Input: part model. Units: mm. Frame: model coordinates. A direction names the side the tool comes from. Coordinates: 2 decimals unless noted, no trailing zeros. Order: outer loops, then holes, each group sorted by start corner. A loop starts at its lowest first (then second) coordinate and runs counter-clockwise, first axis right, second up.
Autodesk Fusion 360 part; units mm, degrees
sketch "Esquisse1" plane through (0, 0, 0) normal (0, 0, 1) x (1, 0, 0)
  line L0 (-10, 4.5) -> (57, 4.5)
  line L1 (57, 4.5) -> (57, -4.5)
  line L2 (57, -4.5) -> (-10, -4.5)
  line L3 (-10, -4.5) -> (-10, 4.5)
  dimension "d1" = 67
  dimension "d2" = 9
  dimension "d3" = 10
  dimension "d4" = 4.5
extrude "Extrusion1" add sketch "Esquisse1" along normal blind 1.6
sketch "Esquisse2" plane through (0, 0, 1.6) normal (0, 0, 1) x (-1, 0, 0)
  line L0 (10, 4.5) -> (-57, 4.5)
  line L1 (-57, 4.5) -> (-57, -4.5)
  line L2 (-57, -4.5) -> (10, -4.5)
  line L3 (10, -4.5) -> (10, 4.5)
  circle A0 centre (0, 0) radius 3.5
  arc A1 (-35.2136, 4.5) -> (-35.2135, -4.5007) centre (0, 0) ccw
  arc A2 (-36.2215, 4.5) -> (-36.2215, -4.5) centre (0, 0) ccw
  line L4 (-35.2135, -4.5007) -> (-36.2215, -4.5)
  line L5 (-35.2135, -4.5007) -> (-36.2215, -4.5)
  line L6 (-35.2136, 4.5) -> (-36.2215, 4.5)
  circle A3 centre (0, 0) radius 2.8
  dimension "d7" = 7
  dimension "d8" = 35.5
  dimension "d9" = 36.5
  dimension "d10" = 5.6
extrude "Extrusion2" add sketch "Esquisse2" along normal blind 12 contours L0 L2 A1 A2 L4 L5 L6
extrude "Extrusion3" add sketch "Esquisse2" along normal blind 12 contours A0
sketch "Esquisse3" plane through (0, 0, 13.6) normal (0, 0, 1) x (-1, 0, 0)
  circle A0 centre (0, 0) radius 2.8
  circle A1 centre (0, 0) radius 3.5
  line L0 (2.0235, -2.7693) -> (-1.9765, -2.7693)
  line L1 (-1.9765, -2.7693) -> (-1.9765, -2.0693)
  line L2 (-1.9765, -2.0693) -> (2.0235, -2.0693)
  line L3 (2.0235, -2.0693) -> (2.0235, -2.7693)
  dimension "d15" = 4
  dimension "d16" = 0.7
extrude "Extrusion4" add sketch "Esquisse3" against normal blind 12.2 contours A0 L0 L1 L2
sketch "Esquisse4" plane through (0, 0, 1.6) normal (0, 0, 1) x (-1, 0, 0)
  circle A0 centre (-57.5342, 10.9) radius 10.7703
  circle A1 centre (-57.5342, -10.9) radius 10.7705
  dimension "d19" = 21.5407
  dimension "d20" = 21.541
  dimension "d21" = 10.9
  dimension "d22" = 10.9
  dimension "d23" = 57.5342
  dimension "d24" = 57.5342
extrude "Extrusion5" cut sketch "Esquisse4" against normal blind 2
fillet "Congé1" radius 1 1 edges at (3.2631, -1.2657, 1.6)
fillet "Congé2" radius 1 2 edges at (35.5, 0, 1.6) (36.5, 0, 1.6)
equation "d23 = 50.53419 mm + 7 mm"
equation "d24 = 50.53419 mm + 7 mm"
Item 1: Ray query, probe 1 along X at (y, z) = (0, 4.5); probe 2 along Y at (x, z) = (0, 8.25); probe 3 along X at (y, z) = (-1.25, 2). Return the intervals inside material, ascending.
Response values:
probe 1: x = -3.5 to -2.8, 2.8 to 3.5, 35.5 to 36.5
probe 2: y = -3.5 to -2.8, 2.8 to 3.5
probe 3: x = -3.48 to -2.51, 2.51 to 3.48, 35.28 to 36.68
Item 2: Cut plane B-B on x = 29. Return loops of the section in (y, z), then the cut area to 3 significant figures.
Response values:
outline: (-4.5, 0) - (4.5, 0) - (4.5, 1.6) - (-4.5, 1.6) - close
area: 14.4 mm2
Item 3: Draft query along X for faces 6 (the face through (-3.233, -1.341, 8.023)), 7 (the face through (23, 0, 0)), 8 (the face through (52.5, -1.38, 0.81)). Return one class per face: pulls with the +X half, pulls with the -X half, needs draft (parallel to the pull), parting line crosses it, or undercut.
Response values:
face 6: undercut
face 7: needs draft
face 8: pulls with the +X half
Item 4: Access query for faces 1 (the face through (-10, 0, 1)), 2 (the face through (36.5, 0.1, 8)), 3 (the face through (0, 0, 1.6)), 4 (the face through (52.387, 1.439, 0.811)), 5 (the face through (45, 0, 1.6)). Directions: +Z, -Z, +X, -X, +Y, -Y. A direction counts if a zero-diameter tool reaches every point of the face in a straight line with its end or side. Return the directions, or none.
Response values:
face 1: +Z, -Z, -X, +Y, -Y
face 2: +Z, +X
face 3: +Z
face 4: +Z, -Z, +X, +Y
face 5: +Z, +X, +Y, -Y
Item 5: Cut plane A-A on z = 13. Return loops of the section in (x, y), then the cut area to 3 significant figures.
Response values:
outline: circle Ø7 at (0, 0); (35.21, -4.5) - (36.22, -4.5) arc R36.5 ccw to (36.22, 4.5) - (35.21, 4.5) arc R35.5 cw to start; hole circle Ø5.6 at (0, 0)
area: 22.9 mm2
Item 6: Pin query (flat end, axial travel): pin 1 Ø5 at (x, y) = (0, 0) entering from +Z; pin 2 Ø8 at (x, z) = (39.5, 9.5) entering from +Y; pin 3 Ø1 at (y, z) = (2.5, 7) entering from +X; pin 4 Ø1.5 at (x, z) = (32.5, 7.5) entering from -Y. Return the tip coordinate at first contact, or that it passes through.
Response values:
pin 1: stops at z = 1.6
pin 2: stops at y = 4.5
pin 3: stops at x = 36.45
pin 4: passes through
